```python
from build123d import *

# Parameters (mm, degrees)
BOSS_EXTRUDE1_DEPTH = 20
SKETCH2_R           = 2.75
CUT_EXTRUDE1_DEPTH  = 20
SKETCH3_R           = 2.75
CUT_EXTRUDE2_DEPTH  = 20
BOSS_EXTRUDE2_DEPTH = 4.5
BOSS_EXTRUDE3_DEPTH = 4.5
CHAMFER1_SIZE       = 0.25


with BuildPart() as part:
    # Sketch1 → Boss-Extrude1 (new body)
    with BuildSketch(Plane(origin=(0, 0, 0), x_dir=(1, 0, 0), z_dir=(0, 1, 0))):
        Polygon((0, 37), (-10, 37), (-10, 10), (-40, 10), (-40, 0), (0, 0), align=None)
    extrude(amount=BOSS_EXTRUDE1_DEPTH)

    # Sketch2 → Cut-Extrude1 (cut)
    with BuildSketch(Plane.ZY.offset(10)):
        with Locations((-27, 10)):
            Circle(SKETCH2_R)
    extrude(amount=-CUT_EXTRUDE1_DEPTH, mode=Mode.SUBTRACT)

    # Sketch3 → Cut-Extrude2 (cut)
    with BuildSketch(Plane(origin=(0, 0, -10), x_dir=(-1, 0, 0), z_dir=(0, 0, -1))):
        with Locations((30, 10)):
            Circle(SKETCH3_R)
    extrude(amount=-CUT_EXTRUDE2_DEPTH, mode=Mode.SUBTRACT)

    # Sketch4 → Boss-Extrude2 (add)
    with BuildSketch(Plane.XZ):
        Polygon((-40, -10), (-10, -10), (-10, -37), align=None)
    extrude(amount=-BOSS_EXTRUDE2_DEPTH)

    # Sketch5 → Boss-Extrude3 (add)
    with BuildSketch(Plane(origin=(0, 20, 0), x_dir=(1, 0, 0), z_dir=(0, 1, 0))):
        Polygon((-40, 10), (-10, 10), (-10, 37), align=None)
    extrude(amount=-BOSS_EXTRUDE3_DEPTH)

    # Chamfer1
    chamfer1_edges = [part.edges().sort_by_distance(p)[0] for p in [
        (0, 10, 0),
        (-40, 10, 0),
        (-10, 10, -29.75),
        (-20, 20, 0),
        (-27.25, 10, 0),
        (-27.25, 10, -10),
        (-20, 0, 0),
    ]]
    chamfer(chamfer1_edges, length=CHAMFER1_SIZE)


solid = part.part
```
CAD build for the part. Positions are in the model's coordinates, mm. A direction names the side the tool comes from. Round coordinates to 2 decimals unless told otherwise and drop trailing zeros. Order: outer loops, then holes, each group sorted by start corner. A loop starts at its lowest first (then second) coordinate and runs counter-clockwise, first axis right, second up.
Item 1: Saw through at C-C on z = -27. Write the cut outline in (x, y), then the cut area to 3 significant figures.
Item 2: Saw through at A-A on x = -6.5. Write the cut outline in (y, z), then the cut area to 3 significant figures.
Item 3: Probe line 1 along Y through (x, z) = (-30, -17); line 2 along Y through (x, z) = (-30, -5); line 3 along Z through (x, y) = (-17, 10.25). List the from-to ranges inside material, lowest first.
Item 4: Pin check, flat tips, straight feed: pin 1 (6.5 mm diameter, centred on y = 10, z = -27, fed in from -X); pin 2 (4 mm diameter, centred on y = 14.5, z = -28, fed in from -X). Stop position of each tip, or through.
Item 5: Tool access for faces 4 (the face through (-19, 15.5, -18)), 5 (the face through (-24.79, 2.22, -23.69)): list every direction of +Z, -Z, +X, -X, +Y, -Y with a clear straight run to the whole face (end or side of a thin tool).
Item 6: Mould opens along Y. For faces 1 (the face through (-15, 0, -14)), 2 (the face through (-40, 10, -5)), 3 (the face through (-25, 10, -10)) say: pulls with the +Y half, pulls with the -Y half, needs draft (parallel to the pull), parting line crosses it, or undercut.
Item 7: Saw through at B-B on y = 2.5. Write the cut outline in (x, z).
Item 8: Saw through at D-D on x = -30. Write the cut outline in (y, z), then the cut area to 3 significant figures.
Reported:
1. outline: (-21.11, 0) - (0, 0) - (0, 7.25) - (-9.75, 7.25) - (-10, 7) - (-10, 4.5) - (-21.11, 4.5) - close; (-21.11, 15.5) - (-10, 15.5) - (-10, 13) - (-9.75, 12.75) - (0, 12.75) - (0, 20) - (-21.11, 20) - close
1. area: 245 mm2
2. outline: (0, -37) - (20, -37) - (20, -0.25) - (19.75, 0) - (0.25, 0) - (0, -0.25) - close; hole circle Ø5.5 at (10, -27)
2. area: 716 mm2
3. line 1: y = 0 to 4.5, 15.5 to 20
3. line 2: y = 0 to 7.25, 12.75 to 20
3. line 3: z = -10 to 0
4. pin 1: stops at x = -10
4. pin 2: stops at x = -21.92
5. face 4: -Z, -X
5. face 5: -Z, -X, +Y, -Y
6. face 1: pulls with the -Y half
6. face 2: needs draft
6. face 3: undercut
7. outline: (-40, -10) - (-10, -37) - (0, -37) - (0, -0.25) - (-0.25, 0) - (-39.75, 0) - (-40, -0.25) - close
8. outline: (0, -19) - (4.5, -19) - (4.5, -10) - (7, -10) - (7.25, -9.75) - (7.25, -0.25) - (7, 0) - (0.25, 0) - (0, -0.25) - close; (12.75, -9.75) - (13, -10) - (15.5, -10) - (15.5, -19) - (20, -19) - (20, -0.25) - (19.75, 0) - (13, 0) - (12.75, -0.25) - close
8. area: 226 mm2
